Drawing for the job (mm, zero at the part's lowest x, y, z). A direction names the side the tool comes from. Coordinates: 2 decimals unless noted, no trailing zeros. Loops run counter-clockwise (first coordinate to the right, second up) from the corner with the lowest first, then second, coordinate; pieces in that order, holes last. Notation, with made-up numbers: (17.25, 48) - (32.25, 48) arc R14 cw to (32.25, 65) - close; hole circle Ø7 at (59, 9.25). An arc over 180 degrees is marked (long way). Put each result on its own line as item: value.
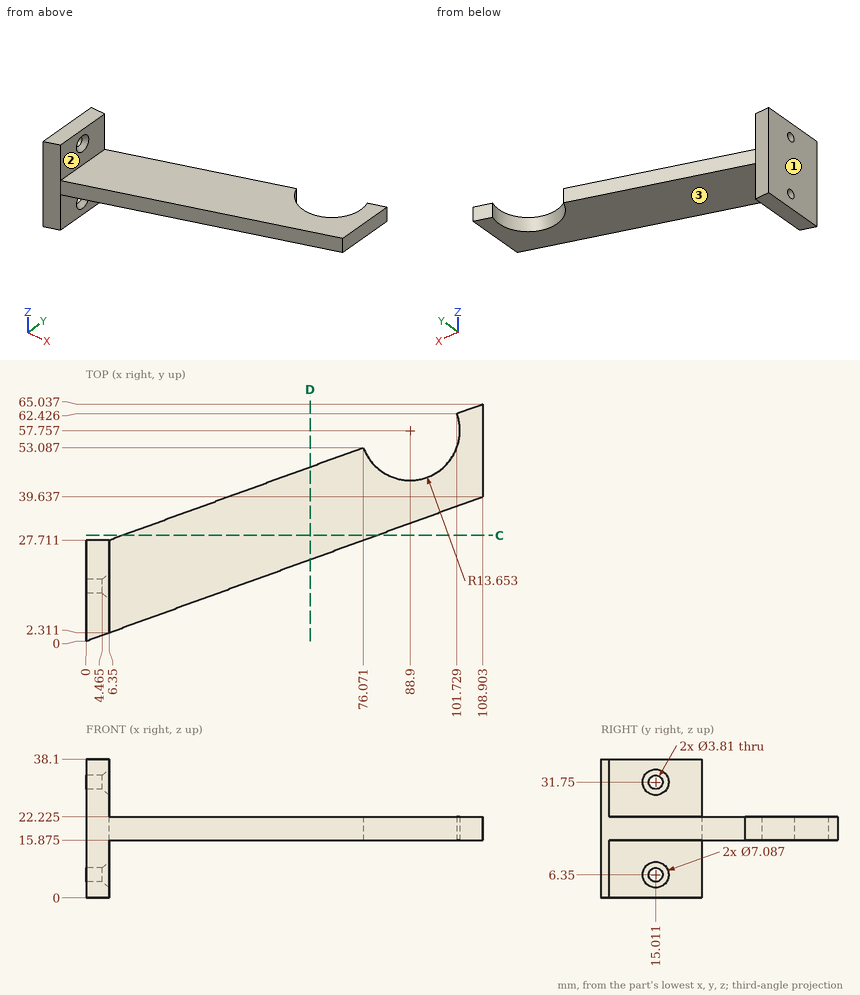
Q1. Tool access for the marked faces 1, 2 and 3: list every direction of +Z, -Z, +X, -X, +Y, -Y with a clear straight run to the whole face (end or side of a thin tool).
Determined:
face 1: +Z, -Z, -X, +Y, -Y
face 2: +Z, +X, +Y, -Y
face 3: -Z, +X, +Y, -Y
Q2. Slice it at C-C, the plane y = 29. Give the cut face in (x, z) (1 decimal), then the cut area to 3 significant figures.
Determined:
outline: (9.9, 15.9) - (79.7, 15.9) - (79.7, 22.2) - (9.9, 22.2) - close
area: 443 mm2
Q3. Slice it at D-D, the plane x = 61.5. Give the cut face in (y, z) (1 decimal).
Determined:
outline: (22.4, 15.9) - (47.8, 15.9) - (47.8, 22.2) - (22.4, 22.2) - close
Q4. Wall check: L1, parallel to Z at x = 62.5, y = 47 (1 decimal); L2, parallel to Y at x = 3.2, z = 6.35 (1 decimal); L3, parallel to X at y = 12.5, z = 11.5. Give the ranges that are in metal, low to high. Write a range as from..to.
Determined:
L1: 15.9..22.2
L2: 1.2..13.1, 16.9..27.7
L3: 0..6.35
Q5. Pin check, flat tips, straight feed: pin 1 Ø5 at (y, z) = (11, 26.5) entering from +X; pin 2 Ø1 at (x, y) = (15.5, 11) entering from +Z (1 decimal); pin 3 Ø6 at (x, z) = (15.5, 16.5) entering from -Y; pin 4 Ø3 at (x, z) = (50, 24) entering from +Y. Stop position of each tip, or through.
Determined:
pin 1: x = 6.35
pin 2: z = 22.2
pin 3: y = 4.55
pin 4: through
